Could you check a few things on this model? Use its own coordinates, in mm. Coordinates: 2 decimals unless noted, no trailing zeros. Write each loop counter-clockwise with the first axis right and the second up, starting at its lowest first coordinate (ties: lowest second). Pieces come first, ordered by that corner, then holes. Notation, with made-up numbers: M -13.75,5 L 35.25,5 A34 cw 35.25,42 Z; hole C -16,-6.75 d8. An arc over 180 degrees is marked long. Answer as CSV lines item,"result". Start each with the question number.
Item 1: I'm going to push flat-ended pins straight in: P1, Ø0.5, axis at x = -53.5, z = 0.5, coming from the +Y side; P2, Ø0.8, axis at x = -51.5, z = 0.5, coming from the -Y side; P3, Ø0.5, axis at y = 85, z = 0.5, coming from the +X side. Where does each tip first touch, or does it pass through?
Item 2: If I drill on line 1 along Y through (x, z) = (-48, 0.9); line 2 along X through (y, z) = (81, 0.3); line 3 along Y through (x, z) = (-46.5, 1.2), over which ranges is the centre line in solid material (lowest first)? Write a range as [from, to].
Item 3: We'd pull the mould along Y, two halves only. Please class faces 1 (the cylindrical face through (45.41, 9.1, 0.81)), 2 (the cylindrical face through (-46.849, 80.854, 0.811)), 3 (the cylindrical face through (-26.367, 5.783, 0.789)), 4 (the cylindrical face through (23.133, 5.783, 0.789)): +Y half, -Y half, draft (parallel to the pull), parting line (faces both ways), or undercut.
Item 4: Suppose I cut it at A-A, the plane z = 1.35. Write out the boundary of the cut face in (x, y).
```python
from build123d import *

# Parameters (mm, degrees)
SKETCH1_R           = 1.1
BOSS_EXTRUDE1_DEPTH = 1.6
FILLET1_R           = 3


with BuildPart() as part:
    # Sketch1 → Boss-Extrude1 (new body)
    with BuildSketch(Plane.XY):
        Polygon((54.006358498, 79.95185693), (44.506358498, 79.95185693), (44.506358498, 85.95185693), (-45.993641502, 85.95185693), (-45.993641502, 79.95185693), (-55.493641502, 79.95185693), (-55.493641502, 9.95185693), (-45.993641502, 9.95185693), (-45.993641502, 3.95185693), (44.506358498, 3.95185693), (44.506358498, 9.95185693), (54.006358498, 9.95185693), align=None)
        with Locations((-25.493641502, 83.45185693)):
            Circle(SKETCH1_R, mode=Mode.SUBTRACT)
        with Locations((24.006358498, 83.45185693)):
            Circle(SKETCH1_R, mode=Mode.SUBTRACT)
        with Locations((24.006358498, 6.45185693)):
            Circle(SKETCH1_R, mode=Mode.SUBTRACT)
        with Locations((-25.493641502, 6.45185693)):
            Circle(SKETCH1_R, mode=Mode.SUBTRACT)
    extrude(amount=BOSS_EXTRUDE1_DEPTH)

    # Fillet1
    fillet1_edges = [part.edges().sort_by_distance(p)[0] for p in [
        (44.506358498, 9.95185693, 0.8),
        (-45.993641502, 9.95185693, 0.8),
        (-45.993641502, 79.95185693, 0.8),
        (44.506358498, 79.95185693, 0.8),
    ]]
    fillet(fillet1_edges, radius=FILLET1_R)


solid = part.part
```
Ans:
1,P1,"stops at y = 79.95"
1,P2,"stops at y = 9.95"
1,P3,"stops at x = 44.51"
2,line 1,"y = [9.78, 80.12]"
2,line 2,"x = [-46.72, 45.23]"
2,line 3,"y = [8.62, 81.28]"
3,face 1,"-Y half"
3,face 2,"+Y half"
3,face 3,"undercut"
3,face 4,"undercut"
4,outline,"M -55.49,9.95 L -48.99,9.95 A3 cw -45.99,6.95 L -45.99,3.95 L 44.51,3.95 L 44.51,6.95 A3 cw 47.51,9.95 L 54.01,9.95 L 54.01,79.95 L 47.51,79.95 A3 cw 44.51,82.95 L 44.51,85.95 L -45.99,85.95 L -45.99,82.95 A3 cw -48.99,79.95 L -55.49,79.95 Z; hole C -25.49,6.45 d2.2; hole C -25.49,83.45 d2.2; hole C 24.01,6.45 d2.2; hole C 24.01,83.45 d2.2"
